Here's the drawing with two shaded views (mm, measured from the low corner). I have some questions. Round coordinates to 2 decimals unless told otherwise and drop trailing zeros. Write each loop counter-clockwise with the first axis right and the second up, starting at its lowest first coordinate (ties: lowest second). Pieces come first, ordered by that corner, then holes. Notation, with made-up numbers: M 59.5,53.25 L 118.5,53.25 A6 cw 118.5,64.25 Z; hole C 3.25,-8.75 d2. An arc over 180 degrees is marked long. Write item = value, one per line. Start each with the question number.
(1) I want a section at C-C (x = 19.5). List the corners of the cut face in (y, z) for me.
(2) I need wall thicknesses on line 1 along Y through (x, z) = (13, 5.5); line 2 along Z through (x, y) = (1.9, 9). Which ranges of each line are inside material? Lowest first, please.
(3) Will this pin go through, and if not, where does the flat tip stop? pin 1 Ø8 at (x, y) = (9, 9) entering from -Z.
(4) I want a section at A-A (y = 8). List the corners of the cut face in (x, z) for me, and give its area (3 significant figures).
(5) I want a section at D-D (z = 9). List the corners of the cut face in (x, y) for me (1 decimal), and give its area (3 significant figures).
(6) If we mould it in two halves opening along Z, with no side actions, what happens to the marked faces 1, 2, 3 and 4? For each: released by +Z, released by -Z, zero draft, split by the parting line, or undercut.
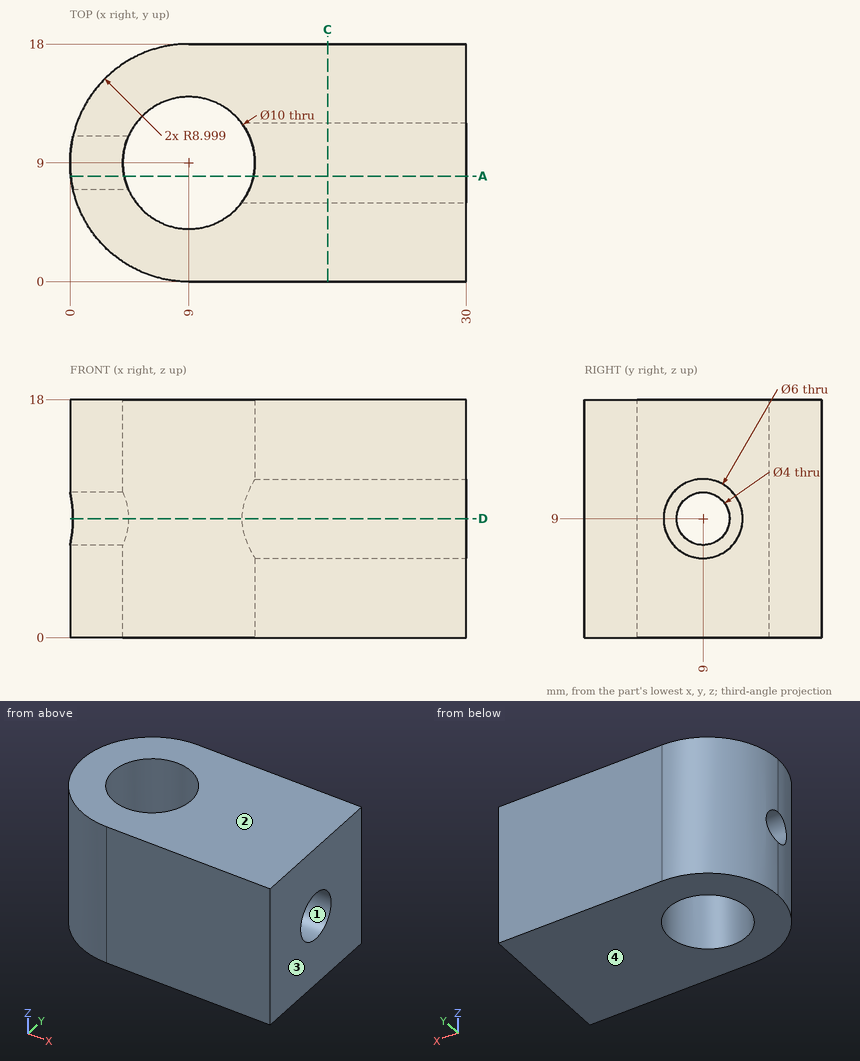
Returned:
q1.outline = M 0,0 L 18,0 L 18,18 L 0,18 Z; hole C 9,9 d6
q2.line_1 = 0 to 6, 12 to 18
q2.line_2 = 0 to 7, 11 to 18
q3.pin_1 = through
q4.outline = M 0.06,0 L 4.1,0 L 4.1,7.27 L 0.06,7.27 Z; M 0.06,10.73 L 4.1,10.73 L 4.1,18 L 0.06,18 Z; M 13.9,0 L 30,0 L 30,6.17 L 13.9,6.17 Z; M 13.9,11.83 L 30,11.83 L 30,18 L 13.9,18 Z
q4.area = 258 mm²
q5.outline = M 0.2,7 A9 ccw 9,0 L 30,0 L 30,6 L 13,6 A5 cw 4.4,7 Z; M 0.2,11 L 4.4,11 A5 cw 13,12 L 30,12 L 30,18 L 9,18 A9 ccw Z
q5.area = 313 mm²
q6.face_1 = undercut
q6.face_2 = released by +Z
q6.face_3 = zero draft
q6.face_4 = released by -Z
